Check sheet for the modelled part. Datum: model origin and axes. Units: mm. A direction names the side the tool comes from. Give positions to 0.01 mm unless a question says otherwise; leave off trailing zeros. Loops run counter-clockwise (first coordinate to the right, second up) from the corner with the lowest first, then second, coordinate; pieces in that order, holes last.
```python
from build123d import *

# Parameters (mm, degrees)
SKETCH1_W                                            = 25
SKETCH1_H                                            = 25
SKETCH1_W_2                                          = 100
SKETCH1_H_2                                          = 75
SKETCH1_R                                            = 12
BOSS_EXTRUDE1_DEPTH                                  = 4
CSK_FOR_M3_HEX_SOCKET_COUNTERSUNK_CAP_SC_D           = 3.4
CSK_FOR_M3_HEX_SOCKET_COUNTERSUNK_CAP_SC_CSINK_D     = 6.72
CSK_FOR_M3_HEX_SOCKET_COUNTERSUNK_CAP_SC_CSINK_ANGLE = 90
M6_CLEARANCE_HOLE2_D                                 = 6.6
FILLET1_R                                            = 5
FILLET2_R                                            = 20


with BuildPart() as part:
    # Sketch1 → Boss-Extrude1 (new body)
    # profile 1 of 3: a face of its own
    with BuildSketch(Plane(origin=(0, 0, 0), x_dir=(1, 0, 0), z_dir=(0, 1, 0))):
        with Locations((-62.5, 25)):
            Rectangle(SKETCH1_W, SKETCH1_H)
    # profile 2 of 3: a face of its own
    with BuildSketch(Plane(origin=(0, 0, 0), x_dir=(1, 0, 0), z_dir=(0, 1, 0))):
        Rectangle(SKETCH1_W_2, SKETCH1_H_2)
        with Locations(Location((0, 0, 0), (0, 0, 270))):
            Circle(SKETCH1_R, mode=Mode.SUBTRACT)
    # profile 3 of 3: a face of its own
    with BuildSketch(Plane(origin=(0, 0, 0), x_dir=(1, 0, 0), z_dir=(0, 1, 0))):
        with Locations((62.5, 25)):
            Rectangle(SKETCH1_W, SKETCH1_H)
    extrude(amount=BOSS_EXTRUDE1_DEPTH)

    # CSK for M3 Hex Socket Countersunk Cap Screw1 (through all)
    with Locations(Plane(origin=(-15.5, 4, 15.5), x_dir=(0, 0, 1), z_dir=(0, 1, 0))):
        with Locations((0, 0), (0, 31), (-31, 31), (-31, 0)):
            CounterSinkHole(CSK_FOR_M3_HEX_SOCKET_COUNTERSUNK_CAP_SC_D / 2, CSK_FOR_M3_HEX_SOCKET_COUNTERSUNK_CAP_SC_CSINK_D / 2, counter_sink_angle=CSK_FOR_M3_HEX_SOCKET_COUNTERSUNK_CAP_SC_CSINK_ANGLE)

    # M6 Clearance Hole2 (through all)
    with Locations(Plane(origin=(0, 0, 0), x_dir=(-1, 0, 0), z_dir=(0, -1, 0))):
        with Locations((62.5, 25), (37.5, -25), (-37.5, -25), (-62.5, 25)):
            Hole(M6_CLEARANCE_HOLE2_D / 2)

    # Fillet1
    fillet1_edges = [part.edges().sort_by_distance(p)[0] for p in [
        (75, 2, -37.5),
        (75, 2, -12.5),
        (50, 2, 37.5),
        (-50, 2, 37.5),
        (-75, 2, -12.5),
        (-75, 2, -37.5),
    ]]
    fillet(fillet1_edges, radius=FILLET1_R)

    # Fillet2
    fillet2_edges = [part.edges().sort_by_distance(p)[0] for p in [
        (50, 2, -12.5),
        (-50, 2, -12.5),
    ]]
    fillet(fillet2_edges, radius=FILLET2_R - 0.0001)  # a hair under: the kernel refuses the full size


solid = part.part
```
(1) Gauge pin test, flat ends, axial feed: pin 1 Ø5.5 at (x, z) = (-15.5, -15.5) entering from +Y; pin 2 Ø5.5 at (x, z) = (-37.5, 25) entering from +Y; pin 3 Ø1.5 at (y, z) = (2.5, 26) entering from +X; pin 4 Ø1.2 at (y, z) = (2.5, 25.5) entering from -X. Record the tip position at first contact, or that the pin passes through.
(2) Material ranges on line 1 (X direction, y = 1.7, z = 15.5); line 2 (Z direction, x = -15.5, y = 0.95); line 3 (X direction, y = 3.1, z = -25), recorded low to high.
(3) Access from +Z, -Z, +X, -X, +Y, -Y to the whole of each face (thin tool, end or side, straight path). Record for faces 1 (the face through (-50, 2, 20)), 2 (the face through (14.85, 1.15, -17.07)).
(4) Section check D-D on y = 1.6. Give the number of separate pieces and of enclosed holes in the cut face, plus the area to 3 significant figures.
(5) Section check B-B on x = -15.5. Record the boundary of the cut face in (y, z), plus the area to 3 significant figures.
(6) Release check for a two-part mould opening along Z. For faces 3 (the face through (50, 2, 20)), 4 (the face through (73.57, 2.03, -36)), 5 (the face through (14, 1.2, 14.7)) record: pulls with the +Z half, pulls with the -Z half, needs draft (parallel to the pull), parting line crosses it, or undercut.
(7) Section check A-A on z = 15.5. Record the boundary of the cut face in (x, y).
(8) Section check C-C on x = 37.5. Record the boundary of the cut face in (y, z), plus the area to 3 significant figures.
Computed values:
1. pin 1: stops at y = 3.39
1. pin 2: passes through
1. pin 3: stops at x = 50
1. pin 4: stops at x = -50
2. line 1: x = -50 to -17.2, -13.8 to 13.8, 17.2 to 50
2. line 2: z = -37.5 to -17.2, -13.8 to 13.8, 17.2 to 37.5
2. line 3: x = -75 to -65.8, -59.2 to 59.2, 65.8 to 75
3. face 1: +Z, -X, +Y, -Y
3. face 2: +Y, -Y
4. separate pieces: 1
4. enclosed holes: 9
4. area: 8,260 mm2
5. outline: (0, -37.5) - (4, -37.5) - (4, -18.86) - (2.34, -17.2) - (0, -17.2) - close; (0, -13.8) - (2.34, -13.8) - (4, -12.14) - (4, 12.14) - (2.34, 13.8) - (0, 13.8) - close; (0, 17.2) - (2.34, 17.2) - (4, 18.86) - (4, 37.5) - (0, 37.5) - close
5. area: 267 mm2
6. face 3: needs draft
6. face 4: pulls with the -Z half
6. face 5: undercut
7. outline: (-50, 0) - (-17.2, 0) - (-17.2, 2.34) - (-18.86, 4) - (-50, 4) - close; (-13.8, 0) - (13.8, 0) - (13.8, 2.34) - (12.14, 4) - (-12.14, 4) - (-13.8, 2.34) - close; (17.2, 0) - (50, 0) - (50, 4) - (18.86, 4) - (17.2, 2.34) - close
8. outline: (0, -37.5) - (4, -37.5) - (4, 21.7) - (0, 21.7) - close; (0, 28.3) - (4, 28.3) - (4, 37.5) - (0, 37.5) - close
8. area: 274 mm2
